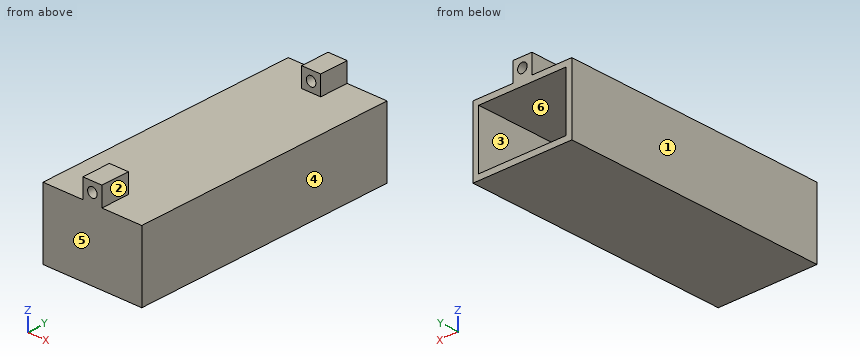
```python
from build123d import *

# Parameters (mm, degrees)
SKETCH1_W               = 52
SKETCH1_H               = 36
BOSS_EXTRUDE1_DEPTH     = 3
BOSS_EXTRUDE2_START     = 3
SKETCH1_3_W             = 52
SKETCH1_3_H             = 36
SKETCH1_3_W_2           = 46
SKETCH1_3_H_2           = 30
BOSS_EXTRUDE2_DEPTH     = 136
SKETCH2_W               = 10
SKETCH2_H               = 15
BOSS_EXTRUDE3_DEPTH     = 10
SKETCH3_R               = 2.5
CUT_EXTRUDE1_DEPTH      = 1
CUT_EXTRUDE1_DEPTH_BACK = 140


with BuildPart() as part:
    # Sketch1 → Boss-Extrude1 (new body)
    with BuildSketch(Plane(origin=(0, 0, 0), x_dir=(1, 0, 0), z_dir=(0, 1, 0))):
        Rectangle(SKETCH1_W, SKETCH1_H)
    extrude(amount=BOSS_EXTRUDE1_DEPTH)

    # Sketch1<3> → Boss-Extrude2 (add)
    with BuildSketch(Plane(origin=(0, 0, 0), x_dir=(1, 0, 0), z_dir=(0, 1, 0)).offset(BOSS_EXTRUDE2_START)):
        Rectangle(SKETCH1_3_W, SKETCH1_3_H)
        Rectangle(SKETCH1_3_W_2, SKETCH1_3_H_2, mode=Mode.SUBTRACT)
    extrude(amount=BOSS_EXTRUDE2_DEPTH)

    # Sketch2 → Boss-Extrude3 (add)
    with BuildSketch(Plane.XY.offset(18)):
        with Locations((0, 131.5)):
            Rectangle(SKETCH2_W, SKETCH2_H)
        with Locations((0, 7.5)):
            Rectangle(SKETCH2_W, SKETCH2_H)
    extrude(amount=BOSS_EXTRUDE3_DEPTH)

    # Sketch3 → Cut-Extrude1 (cut, two sides)
    with BuildSketch(Plane(origin=(0, 139, 0), x_dir=(1, 0, 0), z_dir=(0, 1, 0))) as cut_extrude1_sk:
        with Locations((0, -23)):
            Circle(SKETCH3_R)
    extrude(amount=CUT_EXTRUDE1_DEPTH, mode=Mode.SUBTRACT)
    extrude(cut_extrude1_sk.sketch, amount=-CUT_EXTRUDE1_DEPTH_BACK, mode=Mode.SUBTRACT)


solid = part.part
```
Geometry check sheet. Reference: the model listing, model coordinates, mm. Face numbers are marked on the shaded views. A direction names the side the tool comes from. Coordinates: 2 decimals unless noted, no trailing zeros. Order: outer loops, then holes, each group sorted by start corner. A loop starts at its lowest first (then second) coordinate and runs counter-clockwise, first axis right, second up.
Q1. Sectioned sample at B-B on x = 0. Record the cut outline in (y, z), and give its area (3 significant figures).
Reply:
outline: (0, -18) - (139, -18) - (139, -15) - (3, -15) - (3, 15) - (139, 15) - (139, 20.5) - (124, 20.5) - (124, 18) - (15, 18) - (15, 20.5) - (0, 20.5) - close; (0, 25.5) - (15, 25.5) - (15, 28) - (0, 28) - close; (124, 25.5) - (139, 25.5) - (139, 28) - (124, 28) - close
area: 1,070 mm2
Q2. Sectioned sample at D-D on z = -1. Record the cut outline in (x, y).
Reply:
outline: (-26, 0) - (26, 0) - (26, 139) - (23, 139) - (23, 3) - (-23, 3) - (-23, 139) - (-26, 139) - close
Q3. Sectioned sample at C-C on y = 13. Record the cut outline in (x, z).
Reply:
outline: (-26, -18) - (26, -18) - (26, 18) - (5, 18) - (5, 28) - (-5, 28) - (-5, 18) - (-26, 18) - close; hole (-23, -15) - (23, -15) - (23, 15) - (-23, 15) - close; hole circle Ø5 at (0, 23)
Q4. Sectioned sample at A-A on z = 23. Record the cut outline in (x, y).
Reply:
outline: (-5, 0) - (-2.5, 0) - (-2.5, 15) - (-5, 15) - close; (-5, 124) - (-2.5, 124) - (-2.5, 139) - (-5, 139) - close; (2.5, 0) - (5, 0) - (5, 15) - (2.5, 15) - close; (2.5, 124) - (5, 124) - (5, 139) - (2.5, 139) - close
Q5. Tool access check on the marked faces 1, 2 and 3. Record the directions out of +Z, -Z, +X, -X, +Y, -Y that give a thin tool (end or side, any length) a straight path to the whole face; none if there is none.
Reply:
face 1: +Z, -Z, -X, +Y, -Y
face 2: +Z, +X, +Y, -Y
face 3: +Y
Q6. Thickness scan on probe 1 along Z at (x, y) = (0, 136); probe 2 along X at (y, z) = (135.25, 23); probe 3 along X at (y, z) = (115.5, 12). Record the ranges inside material, lowest first.
Reply:
probe 1: z = -18 to -15, 15 to 20.5, 25.5 to 28
probe 2: x = -5 to -2.5, 2.5 to 5
probe 3: x = -26 to -23, 23 to 26
Q7. Draft check along X on the marked faces 4, 5 and 6. Enter one of: released by +X, released by -X, zero draft, split by the parting line, or undercut.
Reply:
face 4: released by +X
face 5: zero draft
face 6: undercut
Q8. Depth check by flat-ended pin: pin 1 Ø15.5 at (x, y) = (3, 57) entering from +Z; pin 2 Ø3 at (y, z) = (5.5, 21) entering from -X; pin 3 Ø5 at (y, z) = (135, 22) entering from +X. Enter the tip coordinate at first touch or a pass-through.
Reply:
pin 1: stops at z = 18
pin 2: stops at x = -5
pin 3: stops at x = 5
